The listing builds one solid part. Answer for the finished solid, in the listing's coordinates (mm). Give positions to 0.01 mm unless a question says otherwise; leave off trailing zeros. Order: outer loops, then holes, each group sorted by start corner. A loop starts at its lowest first (then second) coordinate and runs counter-clockwise, first axis right, second up. Notation, with made-up numbers: (-19, 83.25) - (12, 83.25) arc R8 cw to (12, 98.25) - close; hole circle Ø9 at (16, 65). An arc over 180 degrees is marked (long way). Answer as a JSON object with one key per item and string values. Group by question number.
Q1. A cutting plane is placed at C-C, the plane z = 3.2. Give the vertices of the cut face in (x, y), and give its area (3 significant figures).
Q2. The mould has two halves that part along Y. Classify faces 1 (the face through (-0.12, -35.25, 2.96)), 2 (the face through (-5.25, -15, 3)), 3 (the face through (2.579, 1.978, 2.958)): released by +Y, released by -Y, zero draft, split by the parting line, or undercut.
Q3. Given pin 1 (3 mm diameter, centred on x = -4, z = 5.5, fed in from -Y), flat-ended and moving along its own axis, determine where the tip first touches the part or whether it passes through.
Q4. A cutting plane is placed at B-B, the plane y = -32. Give the vertices of the cut face in (x, z).
Q5. A cutting plane is placed at A-A, the plane x = 0. Give the vertices of the cut face in (y, z), and give its area (3 significant figures).
Q6. A cutting plane is placed at D-D, the plane x = -2.25. Give the vertices of the cut face in (y, z).
Q7. Consider line 1 (Y direction, x = 0, z = 2.95); line 2 (Y direction, x = 3, z = 5.4); line 3 (X direction, y = -30, z = 0.65). Determine where each line is inside the solid, lowest interval first.
from build123d import *

# Parameters (mm, degrees)
BOSS_EXTRUDE1_DEPTH = 6
SKETCH1_3_R         = 3.25
CUT_EXTRUDE1_DEPTH  = 16


with BuildPart() as part:
    # Sketch1 → Boss-Extrude1 (new body)
    with BuildSketch(Plane.XY):
        with BuildLine():
            Line((-5.25, 0), (-5.25, -30))
            ThreePointArc((-5.25, -30), (0, -35.25), (5.25, -30))
            Line((5.25, -30), (5.25, 0))
            ThreePointArc((5.25, 0), (0, 5.25), (-5.25, 0))
        make_face()
    extrude(amount=BOSS_EXTRUDE1_DEPTH)

    # Sketch1_3 → Cut-Extrude1 (cut)
    with BuildSketch(Plane.XY):
        with Locations(Location((0, -30, 0), (0, 0, 180))):
            Circle(SKETCH1_3_R)
        with Locations(Location((0, 0, 0), (0, 0, 180))):
            Circle(SKETCH1_3_R)
    extrude(amount=CUT_EXTRUDE1_DEPTH, mode=Mode.SUBTRACT)


solid = part.part
Reply:
{
 "1": {"outline": "(-5.25, -30) arc R5.25 ccw to (5.25, -30) - (5.25, 0) arc R5.25 ccw to (-5.25, 0) - close; hole circle Ø6.5 at (0, -30); hole circle Ø6.5 at (0, 0)", "area": "335 mm^2"},
 "2": {"face 1": "released by -Y", "face 2": "zero draft", "face 3": "undercut"},
 "3": {"pin 1": "stops at y = -34.62"},
 "4": {"outline": "(-4.85, 0) - (-2.56, 0) - (-2.56, 6) - (-4.85, 6) - close; (2.56, 0) - (4.85, 0) - (4.85, 6) - (2.56, 6) - close"},
 "5": {"outline": "(-35.25, 0) - (-33.25, 0) - (-33.25, 6) - (-35.25, 6) - close; (-26.75, 0) - (-3.25, 0) - (-3.25, 6) - (-26.75, 6) - close; (3.25, 0) - (5.25, 0) - (5.25, 6) - (3.25, 6) - close", "area": "165 mm^2"},
 "6": {"outline": "(-34.74, 0) - (-32.35, 0) - (-32.35, 6) - (-34.74, 6) - close; (-27.65, 0) - (-2.35, 0) - (-2.35, 6) - (-27.65, 6) - close; (2.35, 0) - (4.74, 0) - (4.74, 6) - (2.35, 6) - close"},
 "7": {"line 1": "y = -35.25 to -33.25, -26.75 to -3.25, 3.25 to 5.25", "line 2": "y = -34.31 to -31.25, -28.75 to -1.25, 1.25 to 4.31", "line 3": "x = -5.25 to -3.25, 3.25 to 5.25"}
}
